Autodesk Inventor part; units mm, degrees
ref_plane "YZ Plane" through (0, 0, 0) normal (1, 0, 0) x (0, 1, 0)
ref_plane "XZ Plane" through (0, 0, 0) normal (0, 1, 0) x (-1, 0, 0)
ref_plane "XY Plane" through (0, 0, 0) normal (0, 0, 1) x (1, 0, 0)
sketch "Sketch1" plane through (0, 0, 0) normal (0, 0, 1) x (1, 0, 0)
  line L0 (0, 0) -> (156.5, 0)
  line L1 (156.5, 0) -> (156.5, 55)
  line L2 (156.5, 55) -> (0, 55)
  line L3 (0, 55) -> (0, 0)
  line L4 (3.269, 40) -> (10, 40)
  line L5 (10, 40) -> (10, 20)
  line L6 (10, 20) -> (3.269, 20)
  line L7 (3.269, 20) -> (3.269, 40)
  line L8 (146.5, 40) -> (153.231, 40)
  line L9 (153.231, 40) -> (153.231, 20)
  line L10 (153.231, 20) -> (146.5, 20)
  line L11 (146.5, 20) -> (146.5, 40)
  line L12 (68.25, 10) -> (88.25, 10)
  line L13 (88.25, 10) -> (88.25, 3.269)
  line L14 (88.25, 3.269) -> (68.25, 3.269)
  line L15 (68.25, 3.269) -> (68.25, 10)
  line L16 (28.25, 55) -> (128.25, 55)
  line L17 (128.25, 55) -> (128.25, 18.269)
  line L18 (128.25, 18.269) -> (28.25, 18.269)
  line L19 (28.25, 18.269) -> (28.25, 55)
  point P0 (3.269, 30)
  point P1 (153.231, 30)
  point P2 (78.25, 18.269)
  point P3 (78.25, 55)
  dimension "d0" = 55
  dimension "d1" = 156.5
  dimension "d2" = 136.5
  dimension "d3" = 6.731
  dimension "d4" = 58.25
  dimension "d5" = 58.25
  dimension "d6" = 20
  dimension "d7" = 3.269
  dimension "d8" = 3.269
  dimension "d25" = 10
  dimension "d26" = 10
  dimension "d28" = 36.731
  dimension "d29" = 100
extrude "Extrusion1" add sketch "Sketch1" along normal blind 6.731 contours L3 L2 L19 L18 L17 L1 L0 | L12 L13 L14 L15
sketch "Sketch2" plane through (0, 0, 6.731) normal (0, 0, 1) x (1, 0, 0)
  line L0 (10, 40) -> (10, 20)
  line L1 (156.5, 55) -> (0, 55)
  line L2 (146.5, 20) -> (146.5, 40)
  point P0 (18.25, 40.769)
  point P1 (138.25, 40.769)
  dimension "d14" = 120
  dimension "d15" = 14.231
  dimension "d16" = -8.25
  dimension "d30" = -8.25
hole "Hole1" at (18.25, 40.769, 6.731) at (138.25, 40.769, 6.731) direction (0, 0, -1) diameter 3.176 end through all
fillet "Fillet1" radius 2 8 edges at (156.5, 55, 3.3655) (0, 55, 3.3655) (0, 0, 3.3655) (156.5, 0, 3.3655) (28.25, 18.269, 3.3655) (28.25, 55, 3.3655) (128.25, 55, 3.3655) (128.25, 18.269, 3.3655)
equation "\"d3\" = THICKB"
equation "\"d4\" = d5"
equation "\"d7\" = d8"
equation "\"d12\" = THICKB"
equation "\"THICKA\" = 3.175"
equation "\"THICKB\" = 6.731"
equation "\"THICKC\" = 12.7"
equation "\"THICKPLY\" = 5"
equation "\"MAGDIA\" = 9.5"
equation "\"BALLDIA\" = 12"
properties part number "Mount_LCD_Back"
The listing builds one solid part. Answer for the finished solid, in the listing's coordinates (mm). A direction names the side the tool comes from. Coordinates: 2 decimals unless noted, no trailing zeros. Write each loop counter-clockwise with the first axis right and the second up, starting at its lowest first coordinate (ties: lowest second). Pieces come first, ordered by that corner, then holes. Notation, with made-up numbers: (32.5, 50.25) - (62.5, 50.25) arc R30 ccw to (62.5, 84.25) - close; hole circle Ø2 at (-27, 66). An arc over 180 degrees is marked (long way). Return JSON: item names as keys, results as strings.
1. This flat-tipped pin is pushed along its axis until it touches: pin 1 Ø3.5 at (x, z) = (101.5, 3) entering from +Y. Where does it stop, or does it pass through?
Final values:
{"pin 1": "y = 18.27"}
2. The part is cut by section C-C on z = 3.75. Determine the outline of the cut face in (x, y).
Final values:
{"outline": "(0, 2) arc R2 ccw to (2, 0) - (154.5, 0) arc R2 ccw to (156.5, 2) - (156.5, 53) arc R2 ccw to (154.5, 55) - (130.25, 55) arc R2 ccw to (128.25, 53) - (128.25, 20.27) arc R2 cw to (126.25, 18.27) - (30.25, 18.27) arc R2 cw to (28.25, 20.27) - (28.25, 53) arc R2 ccw to (26.25, 55) - (2, 55) arc R2 ccw to (0, 53) - close; hole (3.27, 20) - (10, 20) - (10, 40) - (3.27, 40) - close; hole circle Ø3.18 at (18.25, 40.77); hole circle Ø3.18 at (138.25, 40.77); hole (146.5, 20) - (153.23, 20) - (153.23, 40) - (146.5, 40) - close"}
3. For a pull along X with two mould halves and no side action, classify faces 4 (the face through (14, 55, 3)), 5 (the face through (0, 28, 3)), 6 (the face through (3.269, 30, 3)) as +X half, -X half, draft (parallel to the pull), parting line (faces both ways), or undercut.
Final values:
{"face 4": "draft", "face 5": "-X half", "face 6": "undercut"}
4. Which of the six approach directions +Z, -Z, +X, -X, +Y, -Y give full straight-line access (tool end or side, diameter ignored) to faces 1 (the face through (153.231, 30, 3)), 2 (the face through (128.25, 37, 3)), 3 (the face through (77, 0, 3))?
Final values:
{"face 1": "+Z, -Z", "face 2": "+Z, -Z, +Y", "face 3": "+Z, -Z, +X, -X, -Y"}
5. The part is cut by section B-B on y = 30. Determine the outline of the cut face in (x, z).
Final values:
{"outline": "(0, 0) - (3.27, 0) - (3.27, 6.73) - (0, 6.73) - close; (10, 0) - (28.25, 0) - (28.25, 6.73) - (10, 6.73) - close; (128.25, 0) - (146.5, 0) - (146.5, 6.73) - (128.25, 6.73) - close; (153.23, 0) - (156.5, 0) - (156.5, 6.73) - (153.23, 6.73) - close"}
6. Consider line 1 along X through (y, z) = (32, 2.25); line 2 along X through (y, z) = (40.5, 2.75); line 3 along Y through (x, z) = (138.25, 4.5). Determine where each line is inside the solid, lowest interval first.
Final values:
{"line 1": "0 to 3.27, 10 to 28.25, 128.25 to 146.5, 153.23 to 156.5", "line 2": "0 to 16.68, 19.82 to 28.25, 128.25 to 136.68, 139.82 to 156.5", "line 3": "0 to 39.18, 42.36 to 55"}
7. The part is cut by section D-D on x = 93. Determine the outline of the cut face in (y, z).
Final values:
{"outline": "(0, 0) - (18.27, 0) - (18.27, 6.73) - (0, 6.73) - close"}
8. The part is cut by section A-A on x = 138.25. Determine the outline of the cut face in (y, z).
Final values:
{"outline": "(0, 0) - (39.18, 0) - (39.18, 6.73) - (0, 6.73) - close; (42.36, 0) - (55, 0) - (55, 6.73) - (42.36, 6.73) - close"}
